Model file for the job. Use its own axes, mm. Round coordinates to 2 decimals unless told otherwise and drop trailing zeros. Loops run counter-clockwise (first coordinate to the right, second up) from the corner with the lowest first, then second, coordinate; pieces in that order, holes last. Notation, with made-up numbers: M 78.5,50.25 L 128.5,50.25 A28 cw 128.5,83.25 Z; hole C 44.5,-20.75 d1. An arc over 180 degrees is marked long. Use a Markdown table: item, result. Add a question column.
Item 1: Saw through at A-A on z = -6.35. Write the cut outline in (x, y) (3 decimals).
Item 2: Wall check: L1, parallel to X at y = 1.1, z = -19.05. Give the ranges that are in metal, low to high. Write a range as from..to.
Item 3: Saw through at B-B on y = 2.3. Give the number of separate pieces and of enclosed holes in the cut face, then the cut area to 3 significant figures.
Item 4: Pin check, flat tip, straight feed: P1, Ø6.5, axis at x = 0, z = 82.55, coming from the +Y side (3 decimals). Stop position of the tip, or through.
```python
from build123d import *

# Parameters (mm, degrees)
SKETCH2_W           = 38.1
SKETCH2_H           = 203.2
BOSS_EXTRUDE1_DEPTH = 3.175
SKETCH3_R           = 2.794
CUT_EXTRUDE1_DEPTH  = 3.175
LPATTERN1_COUNT     = 16
LPATTERN1_PITCH     = 12.7


with BuildPart() as part:
    # Sketch2 → Boss-Extrude1 (new body)
    with BuildSketch(Plane(origin=(0, 0, 0), x_dir=(1, 0, 0), z_dir=(0, 1, 0))):
        Rectangle(SKETCH2_W, SKETCH2_H)
    extrude(amount=BOSS_EXTRUDE1_DEPTH)

    # Sketch3 → Cut-Extrude1 (cut)
    with BuildSketch(Plane(origin=(0, 3.175, 0), x_dir=(1, 0, 0), z_dir=(0, 1, 0))):
        with Locations(Location((0, -95.25, 0), (0, 0, 270))):
            Circle(SKETCH3_R)
    cut_extrude1 = extrude(amount=-CUT_EXTRUDE1_DEPTH, mode=Mode.SUBTRACT)

    # LPattern1: Cut-Extrude1 ×16
    with Locations(*[(0, 0, -i * LPATTERN1_PITCH) for i in range(1, LPATTERN1_COUNT)]):
        add(cut_extrude1, mode=Mode.SUBTRACT)


solid = part.part
```
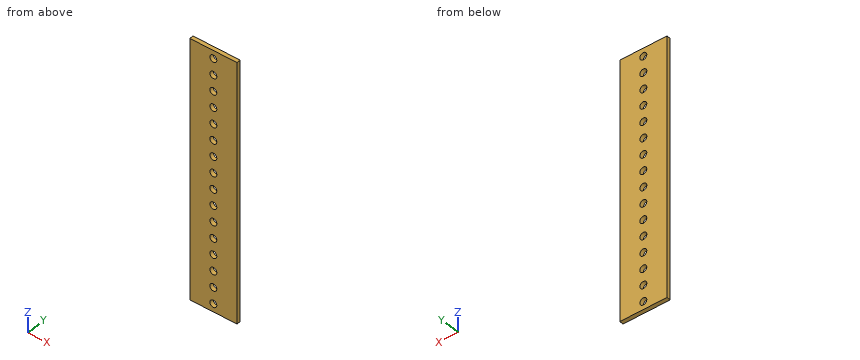
Entries:
| question | item | result |
|---|---|---|
| 1 | outline | M -19.05,0 L -2.794,0 L -2.794,3.175 L -19.05,3.175 Z; M 2.794,0 L 19.05,0 L 19.05,3.175 L 2.794,3.175 Z |
| 2 | L1 | -19.05..-2.79, 2.79..19.05 |
| 3 | separate pieces | 1 |
| 3 | enclosed holes | 16 |
| 3 | area | 7,350 mm2 |
| 4 | P1 | y = 3.175 |
